Study the drawing (mm; zero at the part's minimum x, y, z) and answer. Coordinates: 2 decimals unless noted, no trailing zeros. Write each loop counter-clockwise with the first axis right and the second up, starting at its lowest first coordinate (ties: lowest second). Pieces come first, ordered by that corner, then holes. Notation, with made-up numbers: (55, 48.5) - (103, 48.5) arc R21 ccw to (103, 79.5) - close; hole circle Ø10 at (38, 34.5). An arc over 180 degrees is marked (long way). One line per item, written item: value.
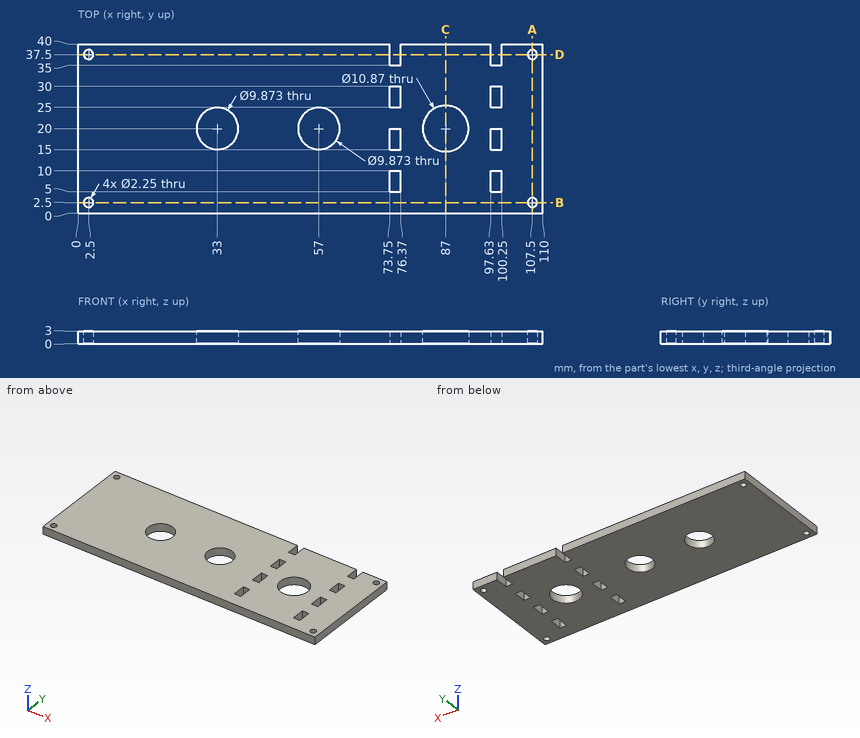
Item 1: Consider probe 1 along Y at (x, z) = (2.5, 0.75) (3 decimals); probe 2 along Y at (x, z) = (99.5, 1.25); probe 3 along X at (y, z) = (28, 1.05). Determine where each line is inside the solid, lowest interval first.
Evaluation:
probe 1: y = 0 to 1.375, 3.625 to 36.375, 38.625 to 40
probe 2: y = 0 to 5, 10 to 15, 20 to 25, 30 to 35
probe 3: x = 0 to 73.75, 76.37 to 97.63, 100.25 to 110
Item 2: Section C-C, the plane x = 87 is taken. Determine the outline of the cut face in (y, z) (3 decimals).
Evaluation:
outline: (0, 0) - (14.565, 0) - (14.565, 3) - (0, 3) - close; (25.435, 0) - (40, 0) - (40, 3) - (25.435, 3) - close
Item 3: Section B-B, the plane y = 2.5 is taken. Determine the outline of the cut face in (x, z) (3 decimals).
Evaluation:
outline: (0, 0) - (1.375, 0) - (1.375, 3) - (0, 3) - close; (3.625, 0) - (106.375, 0) - (106.375, 3) - (3.625, 3) - close; (108.625, 0) - (110, 0) - (110, 3) - (108.625, 3) - close
Item 4: Section A-A, the plane x = 107.5 is taken. Determine the outline of the cut face in (y, z) (3 decimals).
Evaluation:
outline: (0, 0) - (1.375, 0) - (1.375, 3) - (0, 3) - close; (3.625, 0) - (36.375, 0) - (36.375, 3) - (3.625, 3) - close; (38.625, 0) - (40, 0) - (40, 3) - (38.625, 3) - close
Item 5: Section D-D, the plane y = 37.5 is taken. Determine the outline of the cut face in (x, z) (3 decimals), then the cut area to 3 significant figures.
Evaluation:
outline: (0, 0) - (1.375, 0) - (1.375, 3) - (0, 3) - close; (3.625, 0) - (73.75, 0) - (73.75, 3) - (3.625, 3) - close; (76.37, 0) - (97.63, 0) - (97.63, 3) - (76.37, 3) - close; (100.25, 0) - (106.375, 0) - (106.375, 3) - (100.25, 3) - close; (108.625, 0) - (110, 0) - (110, 3) - (108.625, 3) - close
area: 301 mm2
Item 6: Given pin 1 (0.9 mm diameter, centred on y = 27, z = 1, fed in from -X); pin 2 (1.3 mm diameter, centred on x = 75, z = 1, fed in from +Y), each flat-ended and moving along its own axis, determine where each tip first touches the part or whether it passes through.
Evaluation:
pin 1: stops at x = 0
pin 2: stops at y = 35
